Work out the finished part from the listing and answer in its coordinate system (mm). A direction names the side the tool comes from. Coordinates: 2 decimals unless noted, no trailing zeros. Write each loop counter-clockwise with the first axis right and the second up, starting at its lowest first coordinate (ties: lowest second). Pieces come first, ordered by that corner, then holes. Notation, with made-up numbers: (-21.75, -30.75) -> (-10.75, -30.75) arc R32 ccw to (-10.75, 1.25) -> close; hole circle Ø7 at (67.5, 25.5). An arc over 180 degrees is marked (long way). Write each question's results on one line, items separated by ' | '. Start each with the question number.
from build123d import *

# Parameters (mm, degrees)
F0_R     = 0.875
F1_DEPTH = 2
F2_R     = 0.875
F3_DEPTH = 4.001


with BuildPart() as f1:
    # F0 (on Front) → F1 (new body, symmetric)
    with BuildSketch(Plane.XZ):
        with BuildLine():
            ThreePointArc((-10.5, 1.5), (-15, 0), (-10.5, -1.5))
            Line((-10.5, -1.5), (11.1771243445, -1.5))
            ThreePointArc((11.1771243445, -1.5), (10.5, 0), (11.1771243445, 1.5))
            Line((11.1771243445, 1.5), (-10.5, 1.5))
        make_face()
        with Locations((-12.5, 0)):
            Circle(F0_R, mode=Mode.SUBTRACT)
        with BuildLine():
            Line((11.1771243445, 1.5), (11.1771243445, -1.5))
            ThreePointArc((11.1771243445, -1.5), (13.3228756555, -1.8228756555), (14.5, 0))
            ThreePointArc((14.5, 0), (13.3228756555, 1.8228756555), (11.1771243445, 1.5))
        make_face()
        with BuildLine():
            ThreePointArc((11.1771243445, 1.5), (10.5, 0), (11.1771243445, -1.5))
            Line((11.1771243445, -1.5), (11.1771243445, 1.5))
        make_face()
    extrude(amount=F1_DEPTH, both=True)

    # F2 (on face) → F3 (cut, through all)
    with BuildSketch(Plane.XZ.offset(2)):
        with Locations((12.5, 0)):
            Circle(F2_R)
    extrude(amount=-F3_DEPTH, mode=Mode.SUBTRACT)


solid = f1.part
1. Determine the mould class of faces 1 (the face through (-15, 0, 0)), 2 (the face through (0, 2, 0)), 3 (the face through (11.626, -0.028, 0.038)) for opening direction Z: pulls with the +Z half, pulls with the -Z half, needs draft (parallel to the pull), parting line crosses it, or undercut.
2. Find section D-D on x = 12.5. Give the vertices of the cut face in (y, z) (3 decimals), and give its area (3 significant figures).
3. Given pin 1 Ø2 at (x, y) = (-4.5, 0) entering from +Z; pin 2 Ø2 at (y, z) = (-0.5, -0.5) entering from +X; pin 3 Ø1.2 at (x, y) = (-4, 0) entering from -Z, each flat-ended and moving along its own axis, determine where each tip first touches the part or whether it passes through.
4. For faces 4 (the face through (0, 0, -1.5)), 5 (the face through (0, 0, 1.5)), 6 (the face through (0, -2, 0)), determine the directions among +Z, -Z, +X, -X, +Y, -Y from which every point of the face is accessible in a straight line to the end or side of a thin tool.
5. Find section A-A on x = -12.5. Give the vertices of the cut face in (y, z) (3 decimals), and give its area (3 significant figures).
6. Find section B-B on y = 1.6. Give the vertices of the cut face in (x, z) (3 decimals).
7. Find section C-C on z = -0.25. Give the vertices of the cut face in (x, y), and give its area (3 significant figures).
8. Find the intervals of material crossed by L1, parallel to Z at x = -12.5, y = 1 (3 decimals); L2, parallel to Z at x = 12.5, y = 0.5 (3 decimals); L3, parallel to X at y = -1.8, z = 0.4, in increasing order.
Ans:
1) face 1: parting line crosses it | face 2: needs draft | face 3: undercut
2) outline: (-2, -2) -> (2, -2) -> (2, -0.875) -> (-2, -0.875) -> close; (-2, 0.875) -> (2, 0.875) -> (2, 2) -> (-2, 2) -> close | area: 9.00 mm²
3) pin 1: stops at z = 1.5 | pin 2: stops at x = 14.5 | pin 3: stops at z = -1.5
4) face 4: -Z, +Y, -Y | face 5: +Z, +Y, -Y | face 6: +Z, -Z, +X, -X, -Y
5) outline: (-2, -2.5) -> (2, -2.5) -> (2, -0.875) -> (-2, -0.875) -> close; (-2, 0.875) -> (2, 0.875) -> (2, 2.5) -> (-2, 2.5) -> close | area: 13.0 mm²
6) outline: (-10.5, -1.5) -> (11.177, -1.5) arc R2 ccw (long way) to (11.177, 1.5) -> (-10.5, 1.5) arc R2.5 ccw (long way) to start; hole circle Ø1.75 at (-12.5, 0); hole circle Ø1.75 at (12.5, 0)
7) outline: (-14.99, -2) -> (-13.34, -2) -> (-13.34, 2) -> (-14.99, 2) -> close; (-11.66, -2) -> (11.66, -2) -> (11.66, 2) -> (-11.66, 2) -> close; (13.34, -2) -> (14.48, -2) -> (14.48, 2) -> (13.34, 2) -> close | area: 104 mm²
8) L1: z = -2.5 to -0.875, 0.875 to 2.5 | L2: z = -2 to -0.875, 0.875 to 2 | L3: x = -14.97 to -13.28, -11.72 to 11.72, 13.28 to 14.46
